Check sheet for the modelled part. Datum: model origin and axes. Units: mm. A direction names the side the tool comes from. Round coordinates to 2 decimals unless told otherwise and drop trailing zeros. Order: outer loops, then holes, each group sorted by start corner. A loop starts at its lowest first (then second) coordinate and runs counter-clockwise, first axis right, second up. Notation, with made-up numbers: (-11, -2) -> (22, -2) arc R29 ccw to (22, 37) -> close; hole circle Ø8 at (48.5, 72). An arc over 180 degrees is marked (long way). Answer in a Markdown table with one row per item. Add a question column.
1. Depth check by flat-ended pin: P1, Ø1, axis at x = 82.5, y = 3.5, coming from the -Z side; P2, Ø1, axis at y = 4, z = 72.5, coming from the -X side; P3, Ø2.5, axis at y = 4, z = 83, coming from the -X side. Enter the tip coordinate at first touch or a pass-through.
2. Material ranges on L1, parallel to X at y = 0.3, z = 75; L2, parallel to Z at x = 53.5, y = 4; L3, parallel to X at y = 2.5, z = 67, recorded low to high. Write a range as from..to.
3. Draft check along Y on faces 1 (the flat face through (82, 4.2, 68)), 2 (the flat face through (-1, 6, -1)), 3 (the cylindrical face through (78.62, 0.49, -76.85)). Enter one of: +Y half, -Y half, draft (parallel to the pull), parting line (faces both ways), or undercut.
4. Sectioned sample at C-C, the plane z = -58.5. Record the boundary of the cut face in (x, y), then the cut area to 3 significant figures.
5. Sectioned sample at B-B, the plane z = 75. Record the boundary of the cut face in (x, y).
6. Access from +Z, -Z, +X, -X, +Y, -Y to the whole of each face (thin tool, end or side, straight path). Record for faces 4 (the flat face through (76.017, 2, -68)), 5 (the flat face through (22.5, 3, -82)), 6 (the flat face through (82, 2, -53.7)).
7. Sectioned sample at D-D, the plane x = -27. Record the boundary of the cut face in (y, z), then the cut area to 3 significant figures.
8. Sectioned sample at A-A, the plane y = 2.75. Record the boundary of the cut face in (x, z).
```python
from build123d import *

# Parameters (mm, degrees)
SKETCH1_W           = 195
SKETCH1_H           = 170
BOSS_EXTRUDE1_DEPTH = 6
SKETCH2_W           = 90
SKETCH2_H           = 20
CUT_EXTRUDE1_DEPTH  = 130.48841647
FILLET1_R           = 15
SKETCH3_W           = 30
SKETCH3_H           = 6
BOSS_EXTRUDE2_DEPTH = 6
CHAMFER1_SIZE       = 20
SKETCH4_R           = 4
CUT_EXTRUDE2_DEPTH  = 4.2
SKETCH5_W           = 12.3
SKETCH5_H           = 12.3
CUT_EXTRUDE3_DEPTH  = 4.2
SKETCH6_W           = 12.3
SKETCH6_H           = 15.15
CUT_EXTRUDE4_DEPTH  = 3.2


with BuildPart() as part:
    # Sketch1 → Boss-Extrude1 (new body)
    with BuildSketch(Plane(origin=(0, 0, 0), x_dir=(1, 0, 0), z_dir=(0, 1, 0))):
        Rectangle(SKETCH1_W, SKETCH1_H)
    extrude(amount=BOSS_EXTRUDE1_DEPTH)

    # Sketch2 → Cut-Extrude1 (cut, through all)
    with BuildSketch(Plane(origin=(0, 6, 0), x_dir=(1, 0, 0), z_dir=(0, 1, 0))):
        with Locations((-22.5, -75)):
            Rectangle(SKETCH2_W, SKETCH2_H)
        with Locations((-22.5, 75)):
            Rectangle(SKETCH2_W, SKETCH2_H)
    extrude(amount=-CUT_EXTRUDE1_DEPTH, mode=Mode.SUBTRACT)

    # Fillet1
    fillet1_edges = [part.edges().sort_by_distance(p)[0] for p in [
        (-67.5, 3, 65),
        (22.5, 3, 65),
        (-67.5, 3, -65),
        (22.5, 3, -65),
    ]]
    fillet(fillet1_edges, radius=FILLET1_R)

    # Sketch3 → Boss-Extrude2 (add)
    with BuildSketch(Plane(origin=(0, 6, 0), x_dir=(1, 0, 0), z_dir=(0, 1, 0))):
        with Locations((-82.5, 88)):
            Rectangle(SKETCH3_W, SKETCH3_H)
        with Locations((-82.5, -88)):
            Rectangle(SKETCH3_W, SKETCH3_H)
    extrude(amount=-BOSS_EXTRUDE2_DEPTH)

    # Chamfer1
    chamfer1_edges = [part.edges().sort_by_distance(p)[0] for p in [
        (-97.5, 3, -91),
        (-97.5, 3, 91),
    ]]
    chamfer(chamfer1_edges, length=CHAMFER1_SIZE)

    # Sketch4 → Cut-Extrude2 (cut)
    with BuildSketch(Plane.XZ):
        with Locations(Location((82.166666667, -75, 0), (0, 0, 270))):
            Circle(SKETCH4_R)
        with Locations(Location((82.166666667, 75, 0), (0, 0, 90))):
            Circle(SKETCH4_R)
    extrude(amount=-CUT_EXTRUDE2_DEPTH, mode=Mode.SUBTRACT)

    # Sketch5 → Cut-Extrude3 (cut)
    with BuildSketch(Plane.XZ):
        with Locations((82.166666667, 59.85)):
            Rectangle(SKETCH5_W, SKETCH5_H)
        with Locations((82.166666667, -59.85)):
            Rectangle(SKETCH5_W, SKETCH5_H)
    extrude(amount=-CUT_EXTRUDE3_DEPTH, mode=Mode.SUBTRACT)

    # Sketch6 → Cut-Extrude4 (cut)
    with BuildSketch(Plane.XZ.offset(-4.2)):
        with Locations((82.166666667, -73.575)):
            Rectangle(SKETCH6_W, SKETCH6_H)
        with Locations((82.166666667, 73.575)):
            Rectangle(SKETCH6_W, SKETCH6_H)
    extrude(amount=CUT_EXTRUDE4_DEPTH, mode=Mode.SUBTRACT)


solid = part.part
```
Answer key:
| question | item | result |
|---|---|---|
| 1 | P1 | stops at z = -85 |
| 1 | P2 | stops at x = -96.5 |
| 1 | P3 | stops at x = -86.75 |
| 2 | L1 | x = -93.5..-66.64, 21.64..78.17, 86.17..97.5 |
| 2 | L2 | z = -85..85 |
| 2 | L3 | x = -97.5..-59.98, 14.98..76.02, 88.32..97.5 |
| 3 | face 1 | undercut |
| 3 | face 2 | +Y half |
| 3 | face 3 | draft |
| 4 | outline | (-97.5, 0) -> (76.02, 0) -> (76.02, 4.2) -> (88.32, 4.2) -> (88.32, 0) -> (97.5, 0) -> (97.5, 6) -> (-97.5, 6) -> close |
| 4 | area | 1,120 mm² |
| 5 | outline | (-93.5, 0) -> (-66.64, 0) -> (-66.64, 6) -> (-93.5, 6) -> close; (21.64, 0) -> (78.17, 0) -> (78.17, 1) -> (76.02, 1) -> (76.02, 4.2) -> (88.32, 4.2) -> (88.32, 1) -> (86.17, 1) -> (86.17, 0) -> (97.5, 0) -> (97.5, 6) -> (21.64, 6) -> close |
| 6 | face 4 | none |
| 6 | face 5 | -Z, +Y, -Y |
| 6 | face 6 | -Y |
| 7 | outline | (0, -65) -> (6, -65) -> (6, 65) -> (0, 65) -> close |
| 7 | area | 780 mm² |
| 8 | outline | (-97.5, -71) -> (-77.5, -91) -> (-67.5, -91) -> (-67.5, -80) arc R15 cw to (-52.5, -65) -> (7.5, -65) arc R15 cw to (22.5, -80) -> (22.5, -85) -> (97.5, -85) -> (97.5, 85) -> (22.5, 85) -> (22.5, 80) arc R15 cw to (7.5, 65) -> (-52.5, 65) arc R15 cw to (-67.5, 80) -> (-67.5, 91) -> (-77.5, 91) -> (-97.5, 71) -> close; hole (76.02, -81.15) -> (88.32, -81.15) -> (88.32, -53.7) -> (76.02, -53.7) -> close; hole (76.02, 53.7) -> (88.32, 53.7) -> (88.32, 81.15) -> (76.02, 81.15) -> close |
